Model file for the job. Use its own axes, mm. Give positions to 0.01 mm unless a question says otherwise; leave off trailing zeros. Order: outer loops, then holes, each group sorted by start corner. A loop starts at its lowest first (then second) coordinate and runs counter-clockwise, first axis right, second up. Notation, with made-up numbers: M -31.75,-6.5 L 13.25,-6.5 A24 ccw 13.25,17.5 Z; hole C 6.25,50.5 d6. An arc over 180 degrees is marked long. Return JSON: item names as keys, results as strings. Group by question number.
1. Slice it at A-A on y = -0.5. List the corners of the cut face in (x, z) (3 decimals).
2. Wall check: probe 1 along Y at (x, z) = (0, -0.15) (3 decimals); probe 2 along X at (y, z) = (-2, -0.3); probe 3 along Y at (x, z) = (-1, -0.5). Give the ranges that are in metal, low to high. Write a range as [from, to].
3. Slice it at B-B on y = -9. List the corners of the cut face in (x, z) (3 decimals), then the cut area to 3 significant figures.
4. Slice it at C-C on y = -17.5. List the corners of the cut face in (x, z) (3 decimals), then the cut area to 3 significant figures.
5. Pin check, flat tip, straight feed: pin 1 (8.5 mm diameter, centred on x = 0, y = 0, fed in from +Z) (3 decimals). Stop position of the tip, or through.
from build123d import *

# Parameters (mm, degrees)
SKETCH1_R           = 3.175
BOSS_EXTRUDE1_DEPTH = 0.635
SKETCH3_R           = 12.7
CUT_EXTRUDE1_DEPTH  = 239.777071188
CUT_EXTRUDE2_DEPTH  = 2.54


with BuildPart() as part:
    # Sketch1 → Boss-Extrude1 (new, symmetric)
    with BuildSketch(Plane.XY):
        with BuildLine():
            Line((-9.484545184, 0.876942223), (-12.115371852, -27.576693328))
            Line((-12.115371852, -27.576693328), (12.115371852, -27.576693328))
            Line((12.115371852, -27.576693328), (9.484545184, 0.876942223))
            ThreePointArc((9.484545184, 0.876942223), (0, 9.525), (-9.484545184, 0.876942223))
        make_face()
        Circle(SKETCH1_R, mode=Mode.SUBTRACT)
    extrude(amount=BOSS_EXTRUDE1_DEPTH, both=True)

    # Sketch3 → Cut-Extrude1 (cut, through all)
    with BuildSketch(Plane(origin=(-10.234654006, 38.091107641, -227.844114987), x_dir=(-0.9990889360534101, -0.013334766916774946, 0.04053987971048249), z_dir=(-0.04267601884298755, 0.30693794962268295, -0.9507722400749491))):
        Circle(SKETCH3_R)
    extrude(amount=-CUT_EXTRUDE1_DEPTH, mode=Mode.SUBTRACT)

    # Sketch4 → Cut-Extrude2 (cut)
    with BuildSketch(Plane(origin=(0, 0, -0.635), x_dir=(-1, 0, 0), z_dir=(0, 0, -1))):
        with BuildLine():
            Line((-12.115371852, -27.576693328), (12.115371852, -27.576693328))
            Line((12.115371852, -27.576693328), (11.834023856, -24.533781602))
            ThreePointArc((11.834023856, -24.533781602), (10.909017726, -26.125672484), (9.101988814, -25.772969444))
            add(Edge.make_bspline(
                [(9.101988814, -25.772969444), (-0.049020897, -16.134309997), (-9.112527933, -26.125826157)],
                knots=[5.634452132, 5.634452132, 5.634452132, 7.231690845, 7.231690845, 7.231690845], degree=2, weights=[1, 0.697696458, 1]))
            ThreePointArc((-9.112527933, -26.125826157), (-10.927624329, -26.512315749), (-11.869092937, -24.913070304))
            Line((-11.869092937, -24.913070304), (-12.115371852, -27.576693328))
        make_face()
    extrude(amount=-CUT_EXTRUDE2_DEPTH, mode=Mode.SUBTRACT)


solid = part.part
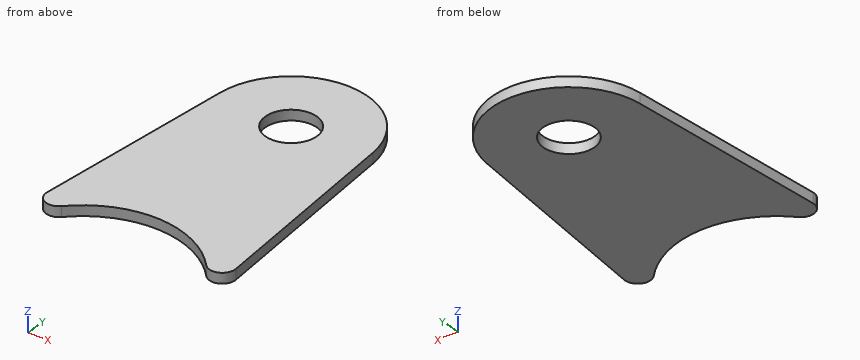
Result:
{
 "1": {"outline": "M -9.612,-0.635 L -3.135,-0.635 L -3.135,0.635 L -9.612,0.635 Z; M 3.135,-0.635 L 9.612,-0.635 L 9.612,0.635 L 3.135,0.635 Z"},
 "2": {"probe 1": "y = [-21.915, -3.175], [3.175, 9.525]", "probe 2": "x = [-9.75, -2.47], [2.47, 9.75]", "probe 3": "y = [-21.94, -3.01], [3.01, 9.47]"},
 "3": {"outline": "M -10.398,-0.635 L 10.398,-0.635 L 10.398,0.635 L -10.398,0.635 Z", "area": "26.4 mm2"},
 "4": {"outline": "M -11.184,-0.635 L 11.184,-0.635 L 11.184,0.635 L -11.184,0.635 Z", "area": "28.4 mm2"},
 "5": {"pin 1": "stops at z = 0.635"}
}
